Read the model definition and answer for the solid it produces. Units are mm, in the model's axes. A direction names the side the tool comes from. Coordinates: 2 decimals unless noted, no trailing zeros. Write each loop counter-clockwise with the first axis right and the second up, starting at its lowest first coordinate (ties: lowest second). Pieces come first, ordered by that corner, then holes.
Item 1: A tool of negligible diameter and unlimited length cuts with its end or side. For faces 4 (the face through (28, 9, -52.5)), 5 (the face through (40, 11.5, -5)), 6 (the face through (23, 14, -58)), from which of +Z, -Z, +X, -X, +Y, -Y can it reach the whole face along a straight path? Write none if from no direction.
Item 2: Each of these flat-tipped pins is pushed along its axis until it touches: P1, Ø4, axis at y = 15.5, z = -12.5, coming from the -X side; P2, Ø3, axis at x = 10, z = -56, coming from the -Y side; P3, Ø12, axis at x = 38, z = -24.5, coming from the +Y side. Where does it stop, or does it pass through?
Item 3: Straight lines are drawn through the part: probe 1 along Z at (x, y) = (40, 8.5); probe 2 along Z at (x, y) = (31.5, 11.75); probe 3 along Y at (x, z) = (44.5, -44.5). For each, find the intervals that lie inside material, in ascending order.
Item 4: Section D-D (z = -5) is taken. Give the vertices of the cut face in (x, y), then the cut area to 3 significant figures.
Item 5: Section A-A (z = -15.75) is taken. Give the vertices of the cut face in (x, y), then the cut area to 3 significant figures.
Item 6: Section B-B (y = 7.25) is taken. Give the vertices of the cut face in (x, z), then the cut area to 3 significant figures.
Item 7: Section C-C (x = 40) is taken. Give the vertices of the cut face in (y, z).
Item 8: Determine the mould class of faces 1 (the face through (28, 5, -32)), 2 (the face through (30, 8, 0)), 3 (the face through (59, 20, -52)) for opening direction Z: released by +Z, released by -Z, zero draft, split by the parting line, or undercut.
from build123d import *

# Parameters (mm, degrees)
SKETCH1_W            = 60
SKETCH1_H            = 62.5
BOSS_EXTRUDE1_DEPTH  = 5
BOSS_EXTRUDE2_DEPTH  = 2.5
BOSS_EXTRUDE3_DEPTH  = 10
BOSS_EXTRUDE4_DEPTH  = 10
SKETCH4_R            = 1.55
CUT_EXTRUDE1_DEPTH   = 10
M5_CLEARANCE_HOLE1_D = 6.4
SKETCH11_W           = 47.107695155
SKETCH11_H           = 10
BOSS_EXTRUDE5_DEPTH  = 2.5


with BuildPart() as part:
    # Sketch1 → Boss-Extrude1 (new body)
    with BuildSketch(Plane(origin=(0, 0, 0), x_dir=(1, 0, 0), z_dir=(0, 1, 0))):
        with Locations((30, 31.25)):
            Rectangle(SKETCH1_W, SKETCH1_H)
    extrude(amount=BOSS_EXTRUDE1_DEPTH)

    # Sketch2 → Boss-Extrude2 (add)
    with BuildSketch(Plane(origin=(60, 0, 0), x_dir=(0, 0, -1), z_dir=(1, 0, 0))):
        with BuildLine():
            Line((0, 20), (0, 5))
            Line((0, 5), (62.5, 5))
            Line((62.5, 5), (62.5, 20))
            Line((62.5, 20), (40.403687781, 20))
            ThreePointArc((40.403687781, 20), (31.25, 15.1), (22.096312219, 20))
            Line((22.096312219, 20), (0, 20))
        make_face()
    extrude(amount=-BOSS_EXTRUDE2_DEPTH)

    # Sketch3 → Boss-Extrude3 (add)
    with BuildSketch(Plane.XY):
        Polygon((57.5, 20), (31.519237886, 5), (57.5, 5), align=None)
    boss_extrude3 = extrude(amount=-BOSS_EXTRUDE3_DEPTH)

    # Sketch8 → Boss-Extrude4 (add)
    with BuildSketch(Plane(origin=(0, 0, 0), x_dir=(-1, 0, 0), z_dir=(0, 0, -1))):
        Polygon((-47.107695155, 14), (-47.107695155, 5), (-33.38717798, 5), (-24.156521096, 5), (0, 5), (0, 14), align=None)
    boss_extrude4 = extrude(amount=BOSS_EXTRUDE4_DEPTH)

    # Mirror1: Boss-Extrude3, Boss-Extrude4 across plane
    add(boss_extrude3.mirror(Plane.XY.offset(-31.25)))
    add(boss_extrude4.mirror(Plane.XY.offset(-31.25)))

    # Sketch4 → Cut-Extrude1 (cut)
    with BuildSketch(Plane(origin=(60, 0, 0), x_dir=(0, 0, -1), z_dir=(1, 0, 0))):
        with Locations((15.75, 10.6)):
            Circle(SKETCH4_R)
        with Locations((46.75, 10.6)):
            Circle(SKETCH4_R)
    extrude(amount=-CUT_EXTRUDE1_DEPTH, mode=Mode.SUBTRACT)

    # M5 Clearance Hole1 (through all)
    with Locations(Plane(origin=(0, 0, 0), x_dir=(-1, 0, 0), z_dir=(0, -1, 0))):
        with Locations((-40, 57.5), (-10, 57.5), (-40, 5), (-10, 5)):
            Hole(M5_CLEARANCE_HOLE1_D / 2)

    # Sketch11 → Boss-Extrude5 (add)
    with BuildSketch(Plane(origin=(0, 14, 0), x_dir=(1, 0, 0), z_dir=(0, 1, 0))):
        with Locations((23.553847578, 57.5)):
            Rectangle(SKETCH11_W, SKETCH11_H)
        with Locations((23.553847578, 5)):
            Rectangle(SKETCH11_W, SKETCH11_H)
    extrude(amount=-BOSS_EXTRUDE5_DEPTH)


solid = part.part
Established:
1. face 4: -X, +Y
1. face 5: -Y
1. face 6: +Z, -Z, -X, +Y
2. P1: stops at x = 57.5
2. P2: stops at y = 11.5
2. P3: stops at y = 5
3. probe 1: z = -62.5 to -60.7, -54.3 to -52.5, -10 to -8.2, -1.8 to 0
3. probe 2: z = -62.5 to -52.5, -10 to 0
3. probe 3: y = 0 to 5
4. outline: (0, 0) - (6.8, 0) - (6.8, 11.5) - (13.2, 11.5) - (13.2, 0) - (36.8, 0) - (36.8, 11.5) - (43.2, 11.5) - (43.2, 0) - (60, 0) - (60, 20) - (57.5, 20) - (47.11, 14) - (0, 14) - close
4. area: 739 mm2
5. outline: (0, 0) - (60, 0) - (60, 9.05) - (57.5, 9.05) - (57.5, 5) - (0, 5) - close; (57.5, 12.15) - (60, 12.15) - (60, 20) - (57.5, 20) - close
5. area: 330 mm2
6. outline: (0, -62.5) - (60, -62.5) - (60, 0) - (0, 0) - (0, -10) - (57.5, -10) - (57.5, -52.5) - (0, -52.5) - close; hole circle Ø6.4 at (10, -57.5); hole circle Ø6.4 at (10, -5); hole circle Ø6.4 at (40, -57.5); hole circle Ø6.4 at (40, -5)
6. area: 1,180 mm2
7. outline: (0, -62.5) - (14, -62.5) - (14, -52.5) - (5, -52.5) - (5, -10) - (14, -10) - (14, 0) - (0, 0) - (0, -1.8) - (11.5, -1.8) - (11.5, -8.2) - (0, -8.2) - (0, -54.3) - (11.5, -54.3) - (11.5, -60.7) - (0, -60.7) - close
8. face 1: undercut
8. face 2: released by +Z
8. face 3: zero draft
